Part model, mm, in its own coordinate system. A direction names the side the tool comes from. Round coordinates to 2 decimals unless told otherwise and drop trailing zeros. Loops run counter-clockwise (first coordinate to the right, second up) from the corner with the lowest first, then second, coordinate; pieces in that order, holes last. Notation, with made-up numbers: M 6,46.25 L 33,46.25 A23 cw 33,83.25 Z; hole C 82,-15.75 d9. An arc over 180 degrees is marked long. Put each result on its own line as item: value. Start each with the question number.
1) Which spindle directions (+Z, -Z, +X, -X, +Y, -Y) get a long thin tool onto all of the face, cutting with end or side? Do faces 3 (the flat face through (12, 152, 0)), 4 (the flat face through (12, 81, 0.2)), 5 (the flat face through (12, 244, 0.2)). Say none if no direction does.
2) Probe line 1 along Y through (x, z) = (22, 2.2); line 2 along Z through (x, y) = (17.5, 15.5); line 3 along X through (y, z) = (164.5, 0.5). List the from-to ranges inside material, lowest first.
3) Slice it at A-A on x = 14.5. Give the cut face in (y, z).
4) Slice it at B-B on y = 88. Give the cut face in (x, z), then the cut area to 3 significant figures.
5) Pull direction Y, two halves, no side cores. Call faces 1 (the flat face through (13, 162, 3.2)), 2 (the flat face through (12, 173, 0.2)): +Y half, -Y half, draft (parallel to the pull), parting line (faces both ways), or undercut.
6) Drop flat-ended pins along their axis: pin 1 Ø0.9 at (x, z) = (19, 2.5) entering from +Y; pin 2 Ø10 at (x, y) = (10, 84) entering from +Z; pin 3 Ø2 at (x, y) = (26.5, 171.5) entering from -Z. Give the stop position or say it passes through.
```python
from build123d import *

# Parameters (mm, degrees)
ESQUISSE1_W      = 25
ESQUISSE1_H      = 300
EXTRUSION1_DEPTH = 0.2
EXTRUSION2_DEPTH = 3


with BuildPart() as part:
    # Esquisse1 → Extrusion1 (new body)
    with BuildSketch(Plane.XY):
        with Locations((12.5, 150)):
            Rectangle(ESQUISSE1_W, ESQUISSE1_H)
    extrude(amount=EXTRUSION1_DEPTH)

    # Esquisse2 → Extrusion2 (add)
    with BuildSketch(Plane.XY.offset(0.2)):
        with BuildLine():
            Line((-0.5, 185.652949425), (25.5, 185.652949425))
            ThreePointArc((25.5, 185.652949425), (28.328427125, 184.48137655), (29.5, 181.652949425))
            Line((29.5, 181.652949425), (29.5, 164.652949425))
            ThreePointArc((29.5, 164.652949425), (28.328427125, 161.8245223), (25.5, 160.652949425))
            Line((25.5, 160.652949425), (-0.5, 160.652949425))
            ThreePointArc((-0.5, 160.652949425), (-3.328427125, 161.8245223), (-4.5, 164.652949425))
            Line((-4.5, 164.652949425), (-4.5, 181.652949425))
            ThreePointArc((-4.5, 181.652949425), (-3.328427125, 184.48137655), (-0.5, 185.652949425))
        make_face()
        with BuildLine():
            Line((-0.5, 182.652949425), (25.5, 182.652949425))
            ThreePointArc((25.5, 182.652949425), (26.207106781, 182.360056206), (26.5, 181.652949425))
            Line((26.5, 181.652949425), (26.5, 164.652949425))
            ThreePointArc((26.5, 164.652949425), (26.207106781, 163.945842644), (25.5, 163.652949425))
            Line((25.5, 163.652949425), (-0.5, 163.652949425))
            ThreePointArc((-0.5, 163.652949425), (-1.207106781, 163.945842644), (-1.5, 164.652949425))
            Line((-1.5, 164.652949425), (-1.5, 181.652949425))
            ThreePointArc((-1.5, 181.652949425), (-1.207106781, 182.360056206), (-0.5, 182.652949425))
        make_face(mode=Mode.SUBTRACT)
    extrude(amount=EXTRUSION2_DEPTH)


solid = part.part
```
Recorded:
1. face 3: -Z, +X, -X, +Y, -Y
1. face 4: +Z, +X, -X, -Y
1. face 5: +Z, +X, -X, +Y
2. line 1: y = 160.65 to 163.65, 182.65 to 185.65
2. line 2: z = 0 to 0.2
2. line 3: x = -4.5 to -1.49, 26.49 to 29.5
3. outline: M 0,0 L 300,0 L 300,0.2 L 185.65,0.2 L 185.65,3.2 L 182.65,3.2 L 182.65,0.2 L 163.65,0.2 L 163.65,3.2 L 160.65,3.2 L 160.65,0.2 L 0,0.2 Z
4. outline: M 0,0 L 25,0 L 25,0.2 L 0,0.2 Z
4. area: 5.00 mm2
5. face 1: draft
5. face 2: undercut
6. pin 1: stops at y = 185.65
6. pin 2: stops at z = 0.2
6. pin 3: stops at z = 0.2
